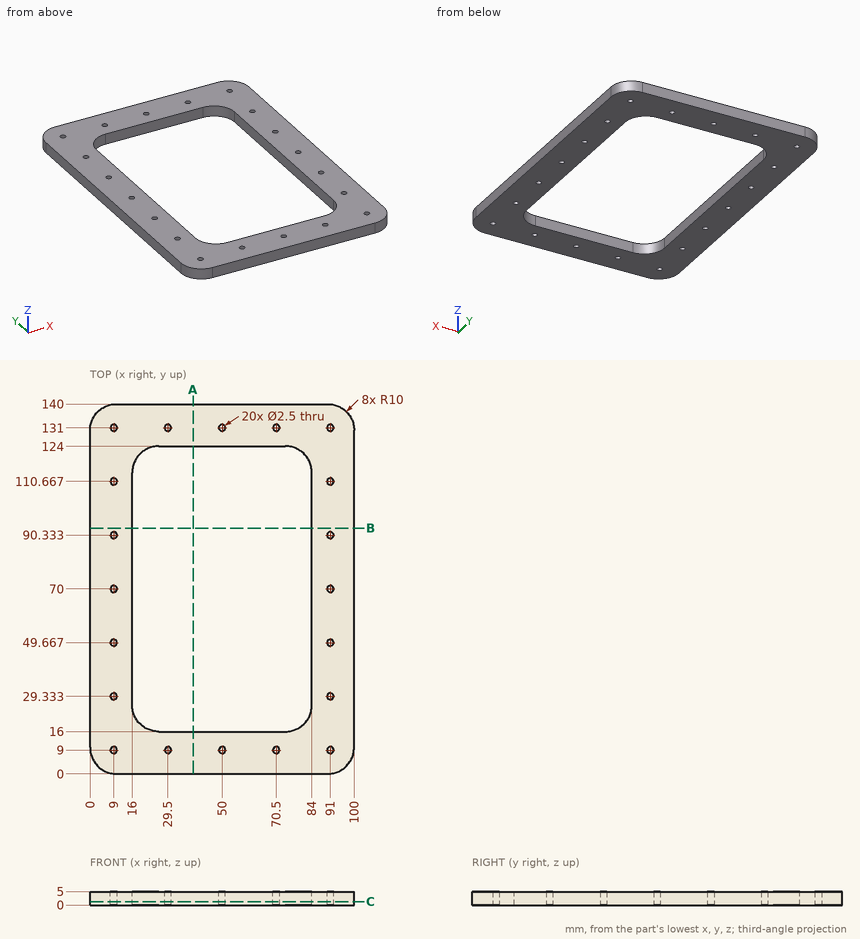
Here's the drawing with two shaded views (mm, measured from the low corner). I have some questions. Round coordinates to 2 decimals unless told otherwise and drop trailing zeros. Loops run counter-clockwise (first coordinate to the right, second up) from the corner with the lowest first, then second, coordinate; pieces in that order, holes last. Notation, with made-up numbers: M 5,6.5 L 42,6.5 A22 ccw 42,28.5 Z; hole C 13.5,-27.75 d2. An arc over 180 degrees is marked long. Answer as CSV lines item,"result".
1) Imagine slicing it at A-A on x = 39. List the corners of the cut face in (y, z) for me.
From the geometry:
outline,"M 0,0 L 16,0 L 16,5 L 0,5 Z; M 124,0 L 140,0 L 140,5 L 124,5 Z"
2) Imagine slicing it at C-C on z = 1.3. Count the separate pieces of the cut face and the enclosed holes in it, and give its area (3 significant figures).
From the geometry:
separate pieces,"1"
enclosed holes,"21"
area,"6,560 mm^2"
3) For pin 1 Ø1.5 at (x, y) = (9, 110.67) entering from +Z; pin 2 Ø3 at (x, y) = (29.5, 131) entering from -Z, each with a flat end and sliding along its axis, tell me the tip position at first contact or that it passes through.
From the geometry:
pin 1,"through"
pin 2,"z = 0"
4) If I drill on probe 1 along Y at (x, z) = (52, 2.8); probe 2 along X at (y, z) = (26, 3.3); probe 3 along Y at (x, z) = (50, 3.5), over which ranges is the centre line in solid material (lowest first)?
From the geometry:
probe 1,"0 to 16, 124 to 140"
probe 2,"0 to 16, 84 to 100"
probe 3,"0 to 7.75, 10.25 to 16, 124 to 129.75, 132.25 to 140"
5) Imagine slicing it at B-B on y = 93. List the corners of the cut face in (x, z) for me, and give its area (3 significant figures).
From the geometry:
outline,"M 0,0 L 16,0 L 16,5 L 0,5 Z; M 84,0 L 100,0 L 100,5 L 84,5 Z"
area,"160 mm^2"
